Print and shaded views of the part. All mm, measured from the part's lowest x, y and z. A direction names the side the tool comes from. Round coordinates to 2 decimals unless told otherwise and drop trailing zeros. Loops run counter-clockwise (first coordinate to the right, second up) from the corner with the lowest first, then second, coordinate; pieces in that order, holes last. Notation, with made-up numbers: (38.25, 13.25) -> (58.25, 13.25) arc R16 cw to (58.25, 41.25) -> close; hole circle Ø9 at (37.25, -22). An arc over 180 degrees is marked (long way). Answer as CSV lines item,"result".
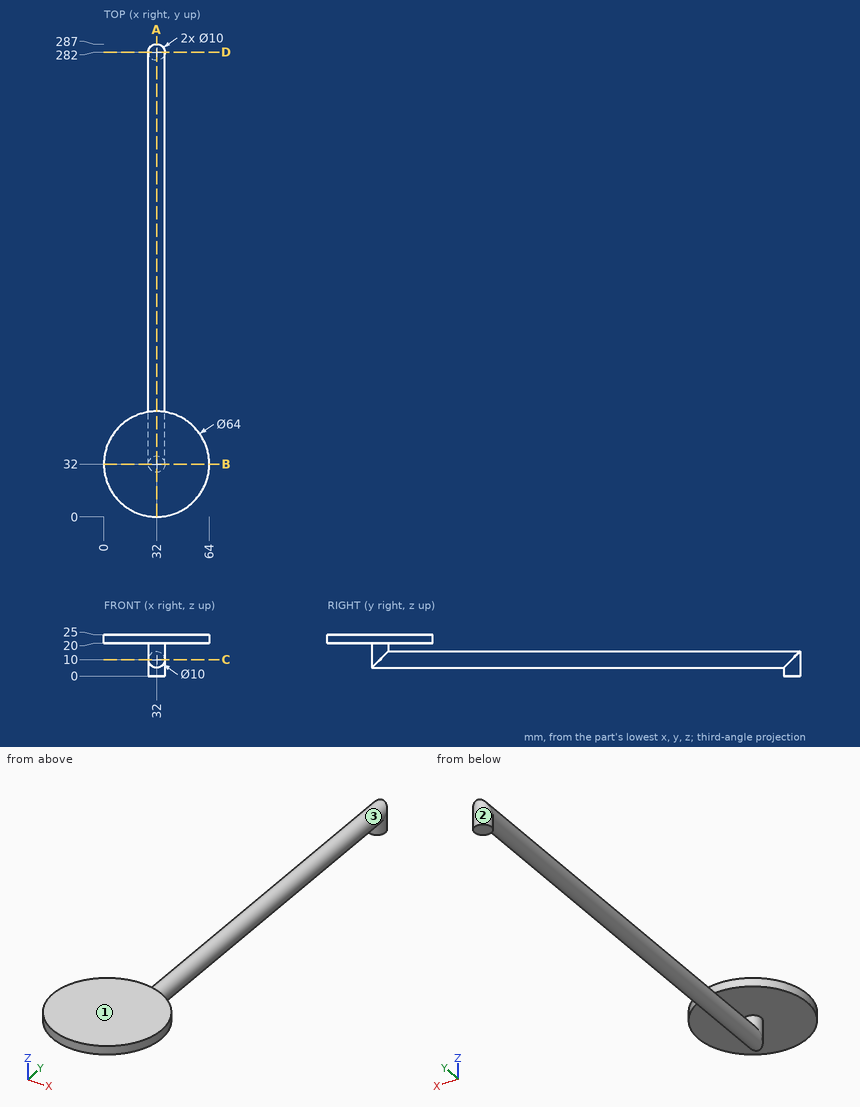
Q1. Saw through at B-B, the plane y = 32. Write the cut outline in (x, z).
Geometry results:
outline,"(0, 20) -> (27, 20) -> (27, 10) arc R5 ccw to (37, 10) -> (37, 20) -> (64, 20) -> (64, 25) -> (0, 25) -> close"
Q2. Drop flat-ended pins along their axis: P1, Ø4, axis at y = 249, z = 5, coming from the -X side; P2, Ø12, axis at y = 100.5, z = 3.5, coming from the +X side; P3, Ø12, axis at x = 41.5, z = 17.5, coming from the +Y side; P4, Ø6, axis at x = 23, y = 213, coming from the -Z side. Give the stop position or say it passes through.
Geometry results:
P1,"x = 28"
P2,"x = 36.97"
P3,"y = 63.74"
P4,"through"
Q3. Saw through at D-D, the plane y = 282. Write the cut outline in (x, z).
Geometry results:
outline,"(27, 0) -> (37, 0) -> (37, 10) arc R5 ccw to (27, 10) -> close"
Q4. Drill centre lines: line 1 along X through (y, z) = (94, 10.75); line 2 along Y through (x, z) = (32.5, 2.75); line 3 along Z through (x, y) = (11.5, 28). Where is each one in solid material? Low to high.
Geometry results:
line 1,"27.06 to 36.94"
line 2,"277.03 to 286.97"
line 3,"20 to 25"
Q5. Saw through at C-C, the plane z = 10. Write the cut outline in (x, y).
Geometry results:
outline,"(27, 32) arc R5 ccw to (37, 32) -> (37, 282) arc R5 ccw to (27, 282) -> close"
Q6. Saw through at A-A, the plane x = 32. Write the cut outline in (y, z), then the cut area to 3 significant figures.
Geometry results:
outline,"(0, 20) -> (27, 20) -> (27, 5) -> (277, 5) -> (277, 0) -> (287, 0) -> (287, 15) -> (37, 15) -> (37, 20) -> (64, 20) -> (64, 25) -> (0, 25) -> close"
area,"3,020 mm2"
Q7. Which spindle directions (+Z, -Z, +X, -X, +Y, -Y) get a long thin tool onto all of the face, cutting with end or side? Do the marked faces 1, 2 and 3. Say none if no direction does.
Geometry results:
face 1,"+Z, +X, -X, +Y, -Y"
face 2,"-Z"
face 3,"none"
